Source: three-view drawing plus pictorial views. Frame: mm from the lowest corner of the part. A direction names the side the tool comes from. Round coordinates to 2 decimals unless told otherwise and drop trailing zeros. Order: outer loops, then holes, each group sorted by start corner. A loop starts at its lowest first (then second) coordinate and runs counter-clockwise, first axis right, second up. Notation, with made-up numbers: (48, 38) -> (92, 38) arc R18 cw to (92, 46) -> close; hole circle Ø2 at (26.25, 89.25). An arc over 180 degrees is marked (long way). Answer as CSV lines item,"result". Start each with the question number.
1) Access query for the marked faces 1 and 2. Directions: +Z, -Z, +X, -X, +Y, -Y. A direction counts if a zero-diameter tool reaches every point of the face in a straight line with its end or side. Return the directions, or none.
2) Section query D-D, the plane x = 24.5. Output: boundary loops of the cut face in (y, z).
3) Section query A-A, the plane y = 12.7. Output: boundary loops of the cut face in (x, z), and give its area (3 significant figures).
4) First-contact query: P1, Ø5, axis at y = 21, z = 13.5, coming from the -X side; P2, Ø13.5, axis at x = 30, z = 9, coming from the -Y side; P3, Ø5, axis at x = 9, z = 10.5, coming from the +Y side; P4, Ø2, axis at x = 15.5, y = 8.5, coming from the +Z side. Flat tips, straight axial feed; report the tip coordinate or a pass-through.
5) Section query C-C, the plane x = 12.7. Output: boundary loops of the cut face in (y, z).
6) Mould query, pull axis Y, two halves, no side actions, for the marked faces 3, 4 and 5. Classes: +Y half, -Y half, draft (parallel to the pull), parting line (faces both ways), or undercut.
7) Section query B-B, the plane z = 2.5. Output: boundary loops of the cut face in (x, y), and give its area (3 significant figures).
8) Line query: L1, parallel to Y at x = 12.5, z = 6.75; L2, parallel to Y at x = 33.5, z = 7.25; L3, parallel to Y at x = 15, z = 5.25. Output: solid intervals per line, ascending.
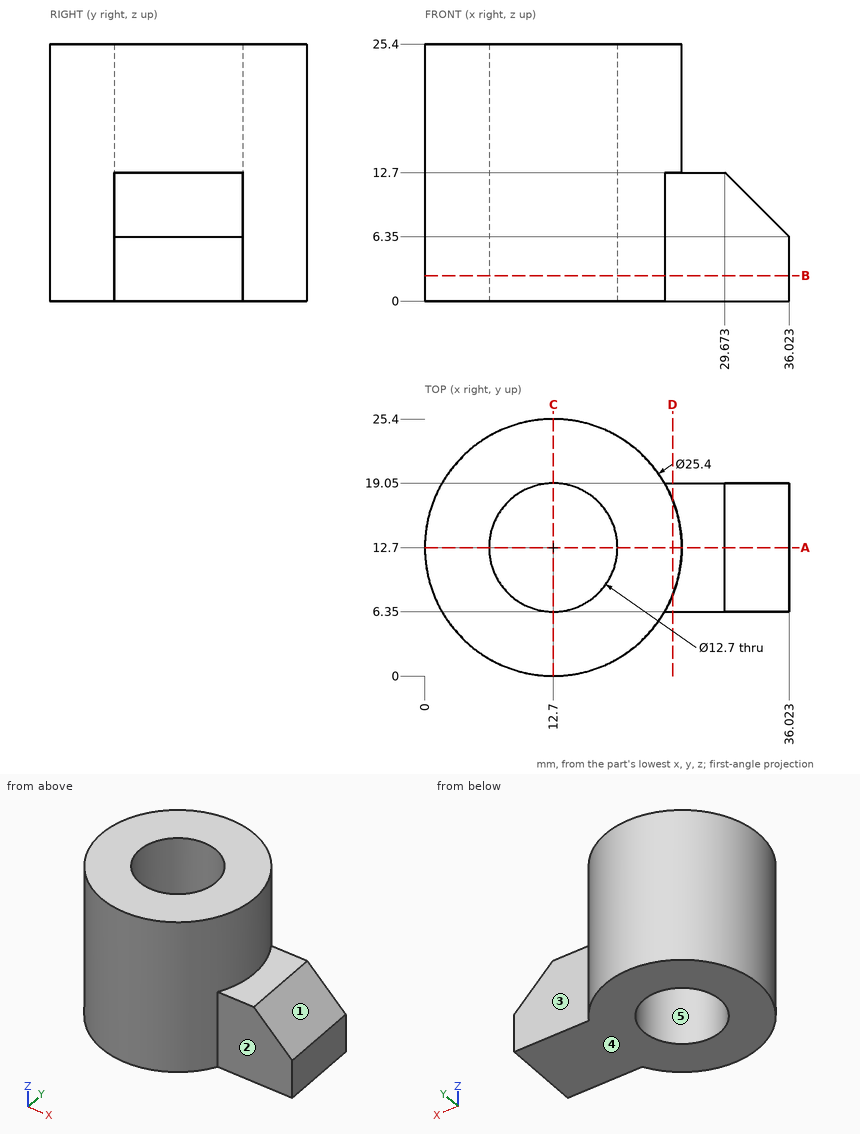
Findings:
1,face 1,"+Z, +X, +Y, -Y"
1,face 2,"+Z, -Z, +X, -Y"
2,outline,"(6.35, 0) -> (19.05, 0) -> (19.05, 12.7) -> (17.4, 12.7) -> (17.4, 25.4) -> (8, 25.4) -> (8, 12.7) -> (6.35, 12.7) -> close"
3,outline,"(0, 0) -> (6.35, 0) -> (6.35, 25.4) -> (0, 25.4) -> close; (19.05, 0) -> (36.02, 0) -> (36.02, 6.35) -> (29.67, 12.7) -> (25.4, 12.7) -> (25.4, 25.4) -> (19.05, 25.4) -> close"
3,area,"437 mm^2"
4,P1,"stops at x = 1.4"
4,P2,"stops at y = 5.63"
4,P3,"stops at y = 25.34"
4,P4,"passes through"
5,outline,"(0, 0) -> (6.35, 0) -> (6.35, 25.4) -> (0, 25.4) -> close; (19.05, 0) -> (25.4, 0) -> (25.4, 25.4) -> (19.05, 25.4) -> close"
6,face 3,"+Y half"
6,face 4,"draft"
6,face 5,"undercut"
7,outline,"(23.7, 6.35) -> (36.02, 6.35) -> (36.02, 19.05) -> (23.7, 19.05) arc R12.7 ccw (long way) to start; hole circle Ø12.7 at (12.7, 12.7)"
7,area,"522 mm^2"
8,L1,"y = 0 to 6.35, 19.05 to 25.4"
8,L2,"y = 6.35 to 19.05"
8,L3,"y = 0.21 to 6.78, 18.62 to 25.19"
